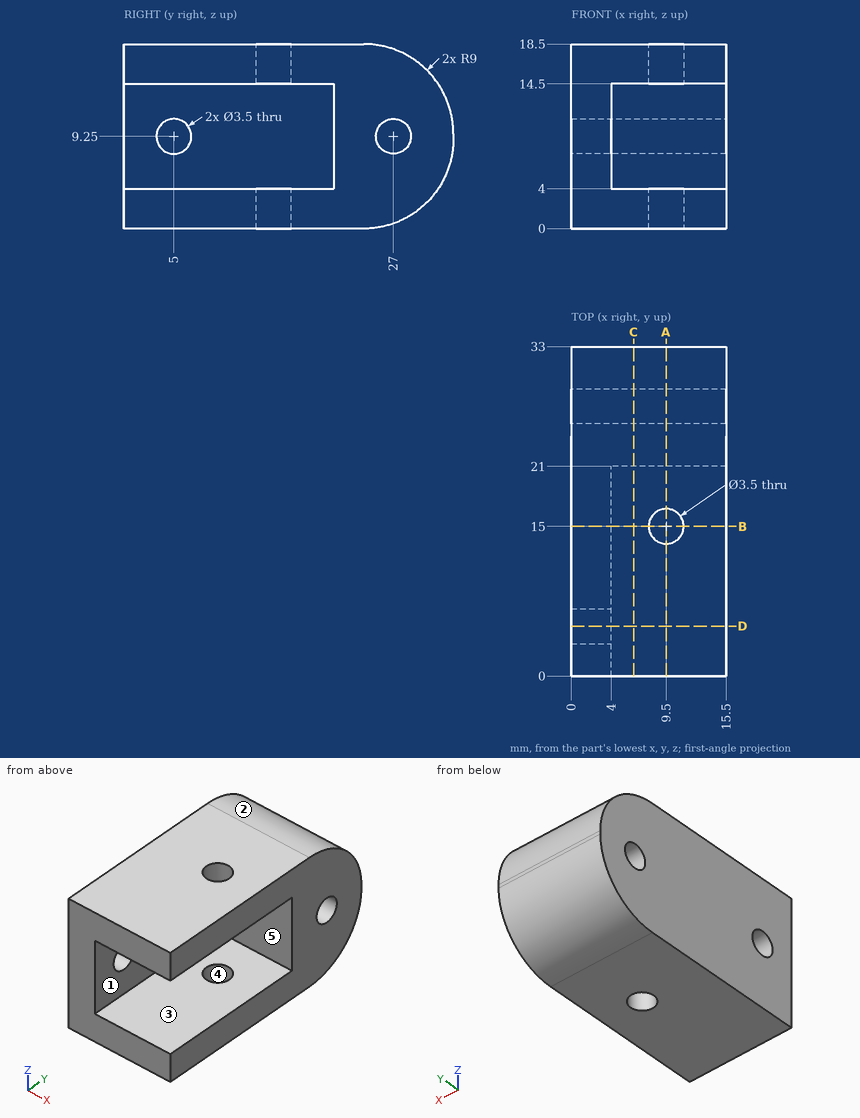
Check sheet for the drawn part. Datum: minimum x, y, z corner. Units: mm. A direction names the side the tool comes from. Give positions to 0.01 mm unless a question says otherwise; leave off trailing zeros. Order: outer loops, then holes, each group sorted by start corner. A loop starts at its lowest first (then second) coordinate and runs counter-clockwise, first axis right, second up. Notation, with made-up numbers: (8, 47) -> (15, 47) arc R10 ccw to (15, 55) -> close; hole circle Ø6 at (-24.75, 23). An arc over 180 degrees is marked (long way). One line per item, written item: value.
(1) Draft check along Y on the marked faces 3, 4 and 5. Enter one of: pulls with the +Y half, pulls with the -Y half, needs draft (parallel to the pull), parting line crosses it, or undercut.
Final values:
face 3: needs draft
face 4: undercut
face 5: pulls with the -Y half
(2) Gauge pin test, flat ends, axial feed: pin 1 (5.5 mm diameter, centred on y = 5, z = 9.25, fed in from -X); pin 2 (5 mm diameter, centred on y = 15.5, z = 10, fed in from +X); pin 3 (1 mm diameter, centred on x = 6, z = 12, fed in from +Y); pin 4 (3 mm diameter, centred on x = 7, z = 10, fed in from -Y). Record the tip position at first contact, or that the pin passes through.
Final values:
pin 1: x = 0
pin 2: x = 4
pin 3: y = 32.77
pin 4: y = 21
(3) Sectioned sample at C-C on x = 6.25. Record the cut outline in (y, z).
Final values:
outline: (0, 0) -> (24, 0) arc R9 ccw to (33, 9) -> (33, 9.5) arc R9 ccw to (24, 18.5) -> (0, 18.5) -> (0, 14.5) -> (21, 14.5) -> (21, 4) -> (0, 4) -> close; hole circle Ø3.5 at (27, 9.25)
(4) Sectioned sample at D-D on y = 5. Record the cut outline in (x, z).
Final values:
outline: (0, 0) -> (15.5, 0) -> (15.5, 4) -> (4, 4) -> (4, 7.5) -> (0, 7.5) -> close; (0, 11) -> (4, 11) -> (4, 14.5) -> (15.5, 14.5) -> (15.5, 18.5) -> (0, 18.5) -> close
(5) Tool access check on the marked faces 1 and 2. Record the directions out of +Z, -Z, +X, -X, +Y, -Y that give a thin tool (end or side, any length) a straight path to the whole face; none if there is none.
Final values:
face 1: +X, -Y
face 2: +Z, +X, -X, +Y
(6) Sectioned sample at B-B on y = 15. Record the cut outline in (x, z), then the cut area to 3 significant figures.
Final values:
outline: (0, 0) -> (7.75, 0) -> (7.75, 4) -> (4, 4) -> (4, 14.5) -> (7.75, 14.5) -> (7.75, 18.5) -> (0, 18.5) -> close; (11.25, 0) -> (15.5, 0) -> (15.5, 4) -> (11.25, 4) -> close; (11.25, 14.5) -> (15.5, 14.5) -> (15.5, 18.5) -> (11.25, 18.5) -> close
area: 138 mm^2
(7) Scan lines: line 1 along Y through (x, z) = (2.2, 9.25); line 2 along Z through (x, y) = (10.5, 16.5); line 3 along Y through (x, z) = (11.5, 9.25). Record each from-to range of solid material in increasing order. Write a range as [from, to].
Final values:
line 1: [0, 3.25], [6.75, 25.25], [28.75, 33]
line 2: [0, 4], [14.5, 18.5]
line 3: [21, 25.25], [28.75, 33]
(8) Sectioned sample at A-A on x = 9.5. Record the cut outline in (y, z).
Final values:
outline: (0, 0) -> (13.25, 0) -> (13.25, 4) -> (0, 4) -> close; (0, 14.5) -> (13.25, 14.5) -> (13.25, 18.5) -> (0, 18.5) -> close; (16.75, 0) -> (24, 0) arc R9 ccw to (33, 9) -> (33, 9.5) arc R9 ccw to (24, 18.5) -> (16.75, 18.5) -> (16.75, 14.5) -> (21, 14.5) -> (21, 4) -> (16.75, 4) -> close; hole circle Ø3.5 at (27, 9.25)
